from build123d import *

# Parameters (mm, degrees)
SKETCH1_R           = 1.5
SKETCH1_W           = 1
SKETCH1_H           = 1
BOSS_EXTRUDE1_DEPTH = 1.6
FILLET1_R           = 1


with BuildPart() as part:
    # Sketch1 → Boss-Extrude1 (new body)
    with BuildSketch(Plane(origin=(0, 0, 0), x_dir=(1, 0, 0), z_dir=(0, 1, 0))):
        with BuildLine():
            ThreePointArc((13.5, 5), (10, 8.5), (6.5, 5))
            Line((6.5, 5), (6.5, -5))
            Line((6.5, -5), (2.5, -5))
            Line((2.5, -5), (2.5, 5))
            ThreePointArc((2.5, 5), (0, 7.5), (-2.5, 5))
            Line((-2.5, 5), (-2.5, -15))
            Line((-2.5, -15), (59.5, -15))
            Line((59.5, -15), (59.5, 10))
            ThreePointArc((59.5, 10), (55, 14.5), (50.5, 10))
            Line((50.5, 10), (50.5, -5))
            Line((50.5, -5), (46.5, -5))
            Line((46.5, -5), (46.5, 10))
            ThreePointArc((46.5, 10), (43, 13.5), (39.5, 10))
            Line((39.5, 10), (39.5, -5))
            Line((39.5, -5), (35.5, -5))
            Line((35.5, -5), (35.5, 10))
            ThreePointArc((35.5, 10), (33, 12.5), (30.5, 10))
            Line((30.5, 10), (30.5, -5))
            Line((30.5, -5), (26.5, -5))
            Line((26.5, -5), (26.5, 5))
            ThreePointArc((26.5, 5), (22, 9.5), (17.5, 5))
            Line((17.5, 5), (17.5, -5))
            Line((17.5, -5), (13.5, -5))
            Line((13.5, -5), (13.5, 5))
        make_face()
        with Locations((10, 5)):
            Circle(SKETCH1_R, mode=Mode.SUBTRACT)
        with Locations((56.5, -12)):
            Circle(SKETCH1_R, mode=Mode.SUBTRACT)
        with Locations((0.5, -12)):
            Circle(SKETCH1_R, mode=Mode.SUBTRACT)
        with Locations((28.5, -12)):
            Circle(SKETCH1_R, mode=Mode.SUBTRACT)
        with Locations((0, 5)):
            Circle(SKETCH1_R, mode=Mode.SUBTRACT)
        with Locations((-0.5, -0.5)):
            Rectangle(SKETCH1_W, SKETCH1_H, mode=Mode.SUBTRACT)
        with Locations((22, 5)):
            Circle(SKETCH1_R, mode=Mode.SUBTRACT)
        with Locations((33, 10)):
            Circle(SKETCH1_R, mode=Mode.SUBTRACT)
        with Locations((55, 10)):
            Circle(SKETCH1_R, mode=Mode.SUBTRACT)
        with Locations((43, 10)):
            Circle(SKETCH1_R, mode=Mode.SUBTRACT)
    extrude(amount=BOSS_EXTRUDE1_DEPTH)

    # Fillet1
    fillet1_edges = [part.edges().sort_by_distance(p)[0] for p in [
        (2.5, 0.8, 5),
        (6.5, 0.8, 5),
        (13.5, 0.8, 5),
        (17.5, 0.8, 5),
        (26.5, 0.8, 5),
        (30.5, 0.8, 5),
        (35.5, 0.8, 5),
        (39.5, 0.8, 5),
        (46.5, 0.8, 5),
        (50.5, 0.8, 5),
        (59.5, 0.8, 15),
        (-2.5, 0.8, 15),
    ]]
    fillet(fillet1_edges, radius=FILLET1_R)


solid = part.part
Verification items for the finished model (mm, model axes). A direction names the side the tool comes from. Coordinates: 2 decimals unless noted, no trailing zeros. Loops run counter-clockwise (first coordinate to the right, second up) from the corner with the lowest first, then second, coordinate; pieces in that order, holes last. Notation, with made-up numbers: (6.25, 75) -> (27.25, 75) arc R30 ccw to (27.25, 110) -> close; hole circle Ø7 at (33, 41.25). An arc over 180 degrees is marked (long way). Answer as a JSON object with one key per item and string values. Group by question number.
Item 1: Sectioned sample at A-A on x = 33. Record the boundary of the cut face in (y, z), plus the area to 3 significant figures.
Item 2: Scan lines: probe 1 along X at (y, z) = (1.15, 12); probe 2 along X at (y, z) = (0.1, -2.5); probe 3 along X at (y, z) = (0.75, -7.75). Record each from-to range of solid material in increasing order.
Item 3: Mould release check, pull along X, two halves, no side actions. Record for faces 3 (the flat face through (6.5, 1, -1)), 4 (the flat face through (59.5, 1, 2)), 5 (the flat face through (28, 1, 15)): +X half, -X half, draft (parallel to the pull), parting line (faces both ways), or undercut.
Item 4: Depth check by flat-ended pin: pin 1 (0.8 mm diameter, centred on y = 1, z = -6.5, fed in from -X) (3 decimals); pin 2 (0.8 mm diameter, centred on x = 15, y = 1, fed in from -Z). Enter the tip coordinate at first touch or a pass-through.
Item 5: Sectioned sample at D-D on y = 0.9. State how many separate pieces and enclosed holes the cut face has, plus the area to 3 significant figures.
Item 6: Sectioned sample at C-C on x = 10. Record the boundary of the cut face in (y, z), plus the area to 3 significant figures.
Item 7: Sectioned sample at B-B on z = 12. Record the boundary of the cut face in (x, y), plus the area to 3 significant figures.
Item 8: Tool access check on faces 1 (the flat face through (17.5, 1, -1)), 2 (the cylindrical face through (31.5, 0.79, -10.07)). Record the directions out of +Z, -Z, +X, -X, +Y, -Y that give a thin tool (end or side, any length) a straight path to the whole face; none if there is none.
Evaluation:
{
 "1": {"outline": "(0, -12.5) -> (1.6, -12.5) -> (1.6, -11.5) -> (0, -11.5) -> close; (0, -8.5) -> (1.6, -8.5) -> (1.6, 15) -> (0, 15) -> close", "area": "39.2 mm²"},
 "2": {"probe 1": "x = -2.5 to -1, 2 to 27, 30 to 55, 58 to 59.5", "probe 2": "x = -2.5 to 2.5, 6.5 to 13.5, 17.5 to 26.5, 30.5 to 35.5, 39.5 to 46.5, 50.5 to 59.5", "probe 3": "x = 7.83 to 12.17, 18.44 to 25.56, 30.5 to 35.5, 39.5 to 46.5, 50.5 to 59.5"},
 "3": {"face 3": "undercut", "face 4": "+X half", "face 5": "draft"},
 "4": {"pin 1": "stops at x = -2.245", "pin 2": "stops at z = 5"},
 "5": {"separate pieces": "1", "enclosed holes": "10", "area": "1,200 mm²"},
 "6": {"outline": "(0, -8.5) -> (1.6, -8.5) -> (1.6, -6.5) -> (0, -6.5) -> close; (0, -3.5) -> (1.6, -3.5) -> (1.6, 15) -> (0, 15) -> close", "area": "32.8 mm²"},
 "7": {"outline": "(-2.5, 0) -> (-1, 0) -> (-1, 1.6) -> (-2.5, 1.6) -> close; (2, 0) -> (27, 0) -> (27, 1.6) -> (2, 1.6) -> close; (30, 0) -> (55, 0) -> (55, 1.6) -> (30, 1.6) -> close; (58, 0) -> (59.5, 0) -> (59.5, 1.6) -> (58, 1.6) -> close", "area": "84.8 mm²"},
 "8": {"face 1": "-Z, +Y, -Y", "face 2": "+Y, -Y"}
}
